from build123d import *

# Parameters (mm, degrees)
F0_W     = 101.6
F0_H     = 146.05
F1_DEPTH = 76.2
F2_T     = -3.81
F4_D     = 3.81


with BuildPart() as f1:
    # F0 (on Top) → F1 (new body)
    with BuildSketch(Plane.XY):
        with Locations((-15.204069, -1.90385)):
            Rectangle(F0_W, F0_H)
    extrude(amount=F1_DEPTH)

    # F2
    f2_openings = [f1.faces().sort_by_distance(p)[0] for p in [
        (-15.204069, -1.90385, 76.2),
    ]]
    offset(amount=F2_T, openings=f2_openings)

    # F4 (through all)
    with Locations(Plane(origin=(0, 71.12115, 0), x_dir=(-1, 0, 0), z_dir=(0, 1, 0))):
        with Locations((59.548918, 72.165899)):
            Hole(F4_D / 2)


solid = f1.part
CAD build for the part. Positions are in the model's coordinates, mm. A direction names the side the tool comes from. Round coordinates to 2 decimals unless told otherwise and drop trailing zeros. Write each loop counter-clockwise with the first axis right and the second up, starting at its lowest first coordinate (ties: lowest second). Pieces come first, ordered by that corner, then holes. Notation, with made-up numbers: (66.25, -19.5) -> (90.25, -19.5) arc R15 cw to (90.25, -3.5) -> close; hole circle Ø3 at (-25, 24.5). An arc over 180 degrees is marked (long way). Answer as a JSON object with one key per item and string values.
(1) Which spindle directions (+Z, -Z, +X, -X, +Y, -Y) get a long thin tool onto all of the face, cutting with end or side? Do faces 1 (the face through (-16, -71.119, 39)), 2 (the face through (-16, -74.929, 38)). Say none if no direction does.
Reported:
{"face 1": "+Z", "face 2": "+Z, -Z, +X, -X, -Y"}
(2) Band-saw the part on B-B, the plane x = -26. List the corners of the cut face in (y, z).
Reported:
{"outline": "(-74.93, 0) -> (71.12, 0) -> (71.12, 76.2) -> (67.31, 76.2) -> (67.31, 3.81) -> (-71.12, 3.81) -> (-71.12, 76.2) -> (-74.93, 76.2) -> close"}
(3) Band-saw the part on C-C, the plane y = -62.5. List the corners of the cut face in (x, z).
Reported:
{"outline": "(-66, 0) -> (35.6, 0) -> (35.6, 76.2) -> (31.79, 76.2) -> (31.79, 3.81) -> (-62.19, 3.81) -> (-62.19, 76.2) -> (-66, 76.2) -> close"}
(4) Probe probe 1 along Y at (x, z) = (31, 59.5); probe 2 along X at (y, z) = (30.5, 59.5); probe 3 along Z at (x, y) = (-13.5, -69). List the from-to ranges inside material, lowest first. Write a range as [from, to].
Reported:
{"probe 1": "y = [-74.93, -71.12], [67.31, 71.12]", "probe 2": "x = [-66, -62.19], [31.79, 35.6]", "probe 3": "z = [0, 3.81]"}
(5) Two-plate mould, pull along X, no slides. Class faces 3 (the face through (35.596, -3, 38)), 4 (the face through (-16, 67.311, 39)), 5 (the face through (-16, 71.121, 38)): +X half, -X half, draft (parallel to the pull), parting line (faces both ways), or undercut.
Reported:
{"face 3": "+X half", "face 4": "undercut", "face 5": "draft"}
(6) Pin check, flat tips, straight feed: P1, Ø12, axis at x = -16.5, y = 49, coming from the +Z side; P2, Ø3.5, axis at x = -59.55, z = 72.17, coming from the -Y side. Stop position of each tip, or through.
Reported:
{"P1": "stops at z = 3.81", "P2": "passes through"}
(7) Band-saw the part on A-A, the plane z = 68. List the corners of the cut face in (x, y), then the cut area to 3 significant figures.
Reported:
{"outline": "(-66, -74.93) -> (35.6, -74.93) -> (35.6, 71.12) -> (-66, 71.12) -> close; hole (-62.19, -71.12) -> (31.79, -71.12) -> (31.79, 67.31) -> (-62.19, 67.31) -> close", "area": "1,830 mm^2"}
